Here's the drawing with two shaded views (mm, measured from the low corner). I have some questions. Coordinates: 2 decimals unless noted, no trailing zeros. Order: outer loops, then holes, each group sorted by start corner. A loop starts at its lowest first (then second) coordinate and runs counter-clockwise, first axis right, second up. Notation, with made-up numbers: (59.25, 0) - (116.25, 0) arc R13 ccw to (116.25, 22) - close; hole circle Ø10 at (-27, 10.25). An arc over 180 degrees is marked (long way). Answer as a JSON object with one key per item and string values. Group by question number.
(1) Please list where these lines run through material, in increasing order: probe 1 along Y at (x, z) = (7, 4.25); probe 2 along Z at (x, y) = (3.25, 10.5); probe 3 along Y at (x, z) = (9, 1.8).
(2) Imagine slicing it at C-C, the plane z = 1.55. Write out the boundary of the cut face in (x, y).
(3) Will these pins go through, and if not, where does the flat tip stop? P1, Ø2.5, axis at x = 7, y = 7, coming from the +Z side; P2, Ø3, axis at x = 4, z = 1, coming from the +Y side.
(4) We'd pull the mould along Y, two halves only. Please class the marked faces 1, 2 and 3: pulls with the +Y half, pulls with the -Y half, needs draft (parallel to the pull), parting line crosses it, or undercut.
(5) Imagine slicing it at D-D, the plane z = 3.35. Write out the boundary of the cut face in (x, y).
(6) Imagine slicing it at A-A, the plane y = 7. Write out the boundary of the cut face in (x, z), and give its area (3 significant figures).
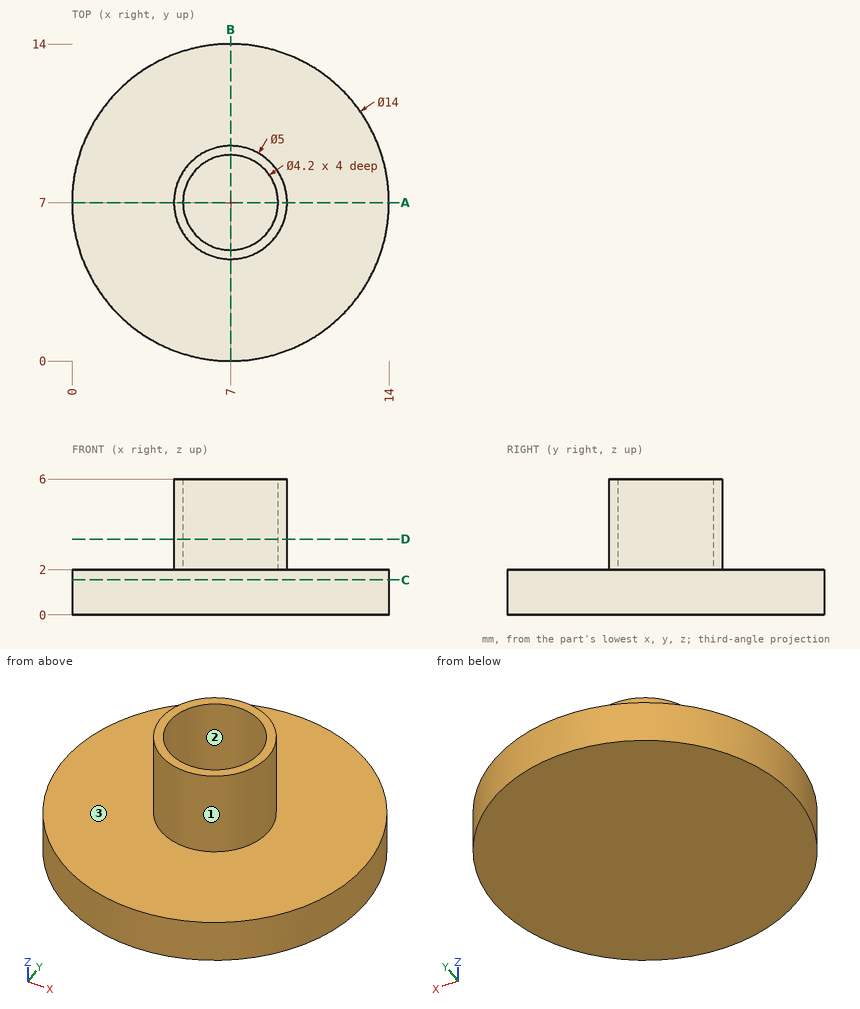
Result set:
{
 "1": {"probe 1": "y = 4.5 to 4.9, 9.1 to 9.5", "probe 2": "z = 0 to 2", "probe 3": "y = 0.29 to 13.71"},
 "2": {"outline": "circle Ø14 at (7, 7)"},
 "3": {"P1": "stops at z = 2", "P2": "stops at y = 13.84"},
 "4": {"face 1": "parting line crosses it", "face 2": "undercut", "face 3": "needs draft"},
 "5": {"outline": "circle Ø5 at (7, 7); hole circle Ø4.2 at (7, 7)"},
 "6": {"outline": "(0, 0) - (14, 0) - (14, 2) - (9.5, 2) - (9.5, 6) - (9.1, 6) - (9.1, 2) - (4.9, 2) - (4.9, 6) - (4.5, 6) - (4.5, 2) - (0, 2) - close", "area": "31.2 mm^2"}
}
